from build123d import *

# Parameters (mm, degrees)
SKETCH1_R           = 21
SKETCH1_R_2         = 1.5
SKETCH1_W           = 4.5
SKETCH1_H           = 4.5
BOSS_EXTRUDE1_DEPTH = 2.5


with BuildPart() as part:
    # Sketch1 → Boss-Extrude1 (new body, symmetric)
    with BuildSketch(Plane(origin=(0, 0, 0), x_dir=(1, 0, 0), z_dir=(0, 1, 0))):
        Circle(SKETCH1_R)
        with Locations((5, 5)):
            Circle(SKETCH1_R_2, mode=Mode.SUBTRACT)
        with Locations((-5, 5)):
            Circle(SKETCH1_R_2, mode=Mode.SUBTRACT)
        with Locations((5, -5)):
            Circle(SKETCH1_R_2, mode=Mode.SUBTRACT)
        with Locations((-5, -5)):
            Circle(SKETCH1_R_2, mode=Mode.SUBTRACT)
        with Locations((-12.5, 12.5)):
            Circle(SKETCH1_R_2, mode=Mode.SUBTRACT)
        with Locations((12.5, 12.5)):
            Circle(SKETCH1_R_2, mode=Mode.SUBTRACT)
        with Locations((12.5, -12.5)):
            Circle(SKETCH1_R_2, mode=Mode.SUBTRACT)
        with Locations((-12.5, -12.5)):
            Circle(SKETCH1_R_2, mode=Mode.SUBTRACT)
        with Locations((12.25, 0)):
            Rectangle(SKETCH1_W, SKETCH1_H, mode=Mode.SUBTRACT)
        with Locations((0, -12.25)):
            Rectangle(SKETCH1_W, SKETCH1_H, mode=Mode.SUBTRACT)
        with Locations((0, 12.25)):
            Rectangle(SKETCH1_W, SKETCH1_H, mode=Mode.SUBTRACT)
        with Locations((-12.25, 0)):
            Rectangle(SKETCH1_W, SKETCH1_H, mode=Mode.SUBTRACT)
    extrude(amount=BOSS_EXTRUDE1_DEPTH, both=True)


solid = part.part
For this review, take the finished solid that the model builds, in its own axes (mm). A direction names the side the tool comes from. Give positions to 0.01 mm unless a question says otherwise; leave off trailing zeros. Order: outer loops, then holes, each group sorted by start corner. A loop starts at its lowest first (then second) coordinate and runs counter-clockwise, first axis right, second up. Notation, with made-up numbers: M -4.5,72 L -0.5,72 A6 cw -0.5,81 Z; hole C 33,56 d9. An arc over 180 degrees is marked long. Answer in a Markdown table with one row per item. Add a question column.
(1) For faces 3 (the face through (12, 0, 2.25)), 4 (the face through (0, 2.5, 0)), list the 3-axis set-ups (+Z, -Z, +X, -X, +Y, -Y) from which the entire face can be reached by the end or side of a thin tool; tool diameter is ignored.
(2) Consider section C-C on y = -1.2. Give the number of separate pieces and of enclosed holes in the cut face, and give its area (3 significant figures).
(3) Mouldability with a two-part tool opening along X and no side actions: class faces 1 (the face through (14.5, 0, 0)), 2 (the face through (0, -2.5, 0)) as +X half, -X half, draft (parallel to the pull), parting line (faces both ways), or undercut.
(4) Wall thickness on probe 1 along X at (y, z) = (0.35, 0); probe 2 along Z at (x, y) = (-12, 1.5); probe 3 along Z at (x, y) = (5, 0.5): over which ranges is each line inside the solid? List them lowest first. Write a range as [from, to].
(5) Consider section A-A on x = 0. State the section outline as (y, z) points, and give its area (3 significant figures).
(6) Consider section B-B on z = 1.5. State the section outline as (x, y) points.
(7) For pin 1 (1.3 mm diameter, centred on x = 11.5, y = -0.5, fed in from -Z); pin 2 (1.3 mm diameter, centred on x = -12, y = -1, fed in from +Z); pin 3 (2 mm diameter, centred on x = 1, y = -0.5, fed in from +Z), all flat-tipped, find the tip position at first contact; note any pin that passes through.
(8) Consider section D-D on z = 12.5. State the section outline as (x, y) points.
Evaluation:
| question | item | result |
|---|---|---|
| 1 | face 3 | +Y, -Y |
| 1 | face 4 | +Z, -Z, +X, -X, +Y |
| 2 | separate pieces | 1 |
| 2 | enclosed holes | 12 |
| 2 | area | 1,250 mm^2 |
| 3 | face 1 | undercut |
| 3 | face 2 | draft |
| 4 | probe 1 | x = [-21, -14.5], [-10, 10], [14.5, 21] |
| 4 | probe 2 | z = [-17.23, -13.91], [-11.09, -2.25], [2.25, 11.09], [13.91, 17.23] |
| 4 | probe 3 | z = [-20.4, -6.5], [-3.5, 3.5], [6.5, 20.4] |
| 5 | outline | M -2.5,-21 L 2.5,-21 L 2.5,-14.5 L -2.5,-14.5 Z; M -2.5,-10 L 2.5,-10 L 2.5,10 L -2.5,10 Z; M -2.5,14.5 L 2.5,14.5 L 2.5,21 L -2.5,21 Z |
| 5 | area | 165 mm^2 |
| 6 | outline | M -20.95,-2.5 L -14.5,-2.5 L -14.5,2.5 L -20.95,2.5 Z; M -10,-2.5 L 10,-2.5 L 10,2.5 L -10,2.5 Z; M 14.5,-2.5 L 20.95,-2.5 L 20.95,2.5 L 14.5,2.5 Z |
| 7 | pin 1 | stops at z = -17.98 |
| 7 | pin 2 | stops at z = 17.67 |
| 7 | pin 3 | stops at z = 21 |
| 8 | outline | M -16.87,-2.5 L -14,-2.5 L -14,2.5 L -16.87,2.5 Z; M -11,-2.5 L -2.25,-2.5 L -2.25,2.5 L -11,2.5 Z; M 2.25,-2.5 L 11,-2.5 L 11,2.5 L 2.25,2.5 Z; M 14,-2.5 L 16.87,-2.5 L 16.87,2.5 L 14,2.5 Z |
